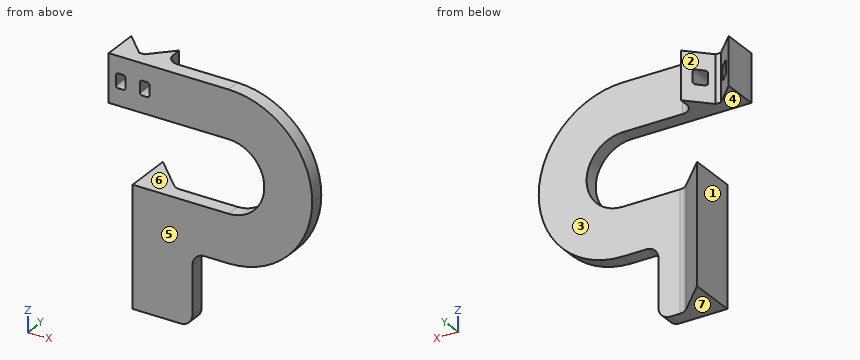
from build123d import *

# Parameters (mm, degrees)
F1_DEPTH = 6
F3_DEPTH = 50
F5_DEPTH = 20
F6_R     = 5
F7_DEPTH = 14.001
F8_R     = 1


with BuildPart() as f1:
    # F0 (on Front) → F1 (new body)
    with BuildSketch(Plane.XZ):
        with BuildLine():
            Line((-10, 15), (8.3772233983, 15))
            ThreePointArc((8.3772233983, 15), (21.2917130661, 29.5803989155), (40, 35))
            Line((40, 35), (-10, 35))
            Line((-10, 35), (-10, 15))
        make_face()
        Polygon((-7, 22), (-7, 25), (-7, 28), (-3, 28), (-3, 25), (-3, 22), align=None, mode=Mode.SUBTRACT)
        Polygon((7, 22), (3, 22), (3, 25), (3, 28), (7, 28), (7, 25), align=None, mode=Mode.SUBTRACT)
        with BuildLine():
            Line((40, -15), (25, -15))
            Line((25, -15), (25, -31.6227766017))
            ThreePointArc((25, -31.6227766017), (32.312255892, -34.1452572187), (40, -35))
            ThreePointArc((40, -35), (64.7487373415, -24.7487373415), (75, 0))
            ThreePointArc((75, 0), (64.7487373415, 24.7487373415), (40, 35))
            ThreePointArc((40, 35), (21.2917130661, 29.5803989155), (8.3772233983, 15))
            Line((8.3772233983, 15), (40, 15))
            ThreePointArc((40, 15), (50.6066017178, 10.6066017178), (55, 0))
            ThreePointArc((55, 0), (50.6066017178, -10.6066017178), (40, -15))
        make_face()
        with BuildLine():
            Line((25, -15), (8.3772233983, -15))
            ThreePointArc((8.3772233983, -15), (15.2512626585, -24.7487373415), (25, -31.6227766017))
            Line((25, -31.6227766017), (25, -15))
        make_face()
        with BuildLine():
            Line((8.3772233983, -15), (0, -15))
            Line((0, -15), (0, -65))
            Line((0, -65), (25, -65))
            Line((25, -65), (25, -35))
            Line((25, -35), (25, -31.6227766017))
            ThreePointArc((25, -31.6227766017), (15.2512626585, -24.7487373415), (8.3772233983, -15))
        make_face()
        with BuildLine():
            ThreePointArc((40, -35), (32.312255892, -34.1452572187), (25, -31.6227766017))
            Line((25, -31.6227766017), (25, -35))
            Line((25, -35), (40, -35))
        make_face()
    extrude(amount=F1_DEPTH)

    # F2 (on face) → F3 (join)
    with BuildSketch(Plane.XY.offset(-15)):
        Polygon((0, 0), (14, 0), (0, 14), align=None)
    extrude(amount=-F3_DEPTH)

    # F4 (on face) → F5 (join, through all)
    with BuildSketch(Plane.XY.offset(35)):
        Polygon((-10, 0), (-1.0710678119, 0), (-10, 8.9289321881), align=None)
        Polygon((1.0710678119, 0), (10, 0), (10, 8.9289321881), align=None)
    extrude(amount=-F5_DEPTH)

    # F6
    f6_edges = [f1.edges().sort_by_distance(p)[0] for p in [
        (25, -3, -35),
        (25, -3, -65),
        (10, 0, 25),
        (14, 0, -40),
    ]]
    fillet(f6_edges, radius=F6_R)

    # F0 (on Front) → F7 (cut, through all)
    with BuildSketch(Plane.XZ):
        Polygon((-7, 28), (-7, 25), (-7, 22), (-3, 22), (-3, 25), (-3, 28), align=None)
        Polygon((3, 25), (3, 22), (7, 22), (7, 25), (7, 28), (3, 28), align=None)
    extrude(amount=-F7_DEPTH, mode=Mode.SUBTRACT)

    # F8
    f8_edges = [f1.edges().sort_by_distance(p)[0] for p in [
        (7, -0.035534, 22),
        (-3, -2.035534, 22),
        (7, -0.035534, 28),
        (-3, -2.035534, 28),
        (-7, -0.035534, 28),
        (3, -2.035534, 28),
        (-7, -0.035534, 22),
        (3, -2.035534, 22),
    ]]
    fillet(f8_edges, radius=F8_R)


solid = f1.part
Input: part model. Units: mm. Frame: model coordinates. Face numbers are marked on the shaded views. A direction names the side the tool comes from. Round coordinates to 2 decimals unless told otherwise and drop trailing zeros. Order: outer loops, then holes, each group sorted by start corner. A loop starts at its lowest first (then second) coordinate and runs counter-clockwise, first axis right, second up. Notation, with made-up numbers: (81, 55.25) - (98, 55.25) arc R15 cw to (98, 74.25) - close; hole circle Ø9 at (-8.5, 83). An arc over 180 degrees is marked (long way). Use a Markdown table: item, result.
1. Access query for the marked faces 1, 2, 3 and 4. Directions: +Z, -Z, +X, -X, +Y, -Y. A direction counts if a zero-diameter tool reaches every point of the face in a straight line with its end or side. Return the directions, or none.
Evaluation:
| item | result |
|---|---|
| face 1 | -Z, -X, +Y, -Y |
| face 2 | +Z, +Y |
| face 3 | +Z, -Z, +X, +Y |
| face 4 | -X, +Y, -Y |
2. Section C-C on z = -57. Return the cut outline in (x, y).
Evaluation:
| item | result |
|---|---|
| outline | (0, -6) - (25, -6) - (25, 0) - (16.07, 0) arc R5 cw to (12.54, 1.46) - (0, 14) - close |
3. Material intervals for probe 1 along Z at (x, y) = (-4, -0.25); probe 2 along Y at (x, z) = (16, 21); probe 3 along Y at (x, z) = (10, -45.5), sorted ascending.
Evaluation:
| item | result |
|---|---|
| probe 1 | 15 to 22, 28 to 35 |
| probe 2 | -6 to 0 |
| probe 3 | -6 to 4 |
4. Section A-A on x = 35.5. Return the cut outline in (y, z), then the cut area to 3 significant figures.
Evaluation:
| item | result |
|---|---|
| outline | (-6, -35) - (0, -35) - (0, -15) - (-6, -15) - close; (-6, 15) - (0, 15) - (0, 35) - (-6, 35) - close |
| area | 240 mm^2 |
5. Section D-D on x = 47.5. Return the cut outline in (y, z).
Evaluation:
| item | result |
|---|---|
| outline | (-6, -34.19) - (0, -34.19) - (0, -12.99) - (-6, -12.99) - close; (-6, 12.99) - (0, 12.99) - (0, 34.19) - (-6, 34.19) - close |
6. First-contact query: pin 1 (2 mm diameter, centred on x = 30.5, z = -36.5, fed in from -Y); pin 2 (4.5 mm diameter, centred on y = -2.5, z = 25.5, fed in from +X); pin 3 (3 mm diameter, centred on y = 6.5, z = 25, fed in from +X); pin 4 (18 mm diameter, centred on x = 39.5, z = -30, fed in from +Y). Flat tips, straight axial feed; report the tip coordinate or a pass-through.
Evaluation:
| item | result |
|---|---|
| pin 1 | through |
| pin 2 | x = 66.16 |
| pin 3 | x = 10 |
| pin 4 | y = 0 |
7. Mould query, pull axis Z, two halves, no side actions, for the marked faces 5, 6 and 7. Classes: +Z half, -Z half, draft (parallel to the pull), parting line (faces both ways), or undercut.
Evaluation:
| item | result |
|---|---|
| face 5 | draft |
| face 6 | undercut |
| face 7 | -Z half |
8. Section B-B on y = -2.5. Return the cut outline in (x, z).
Evaluation:
| item | result |
|---|---|
| outline | (-10, 15) - (40, 15) arc R15 cw to (40, -15) - (0, -15) - (0, -65) - (20, -65) arc R5 ccw to (25, -60) - (25, -40) arc R5 cw to (30, -35) - (40, -35) arc R35 ccw to (40, 35) - (-10, 35) - close; hole (-7, 23) arc R1 ccw to (-6, 22) - (-4, 22) arc R1 ccw to (-3, 23) - (-3, 27) arc R1 ccw to (-4, 28) - (-6, 28) arc R1 ccw to (-7, 27) - close; hole (3, 23) arc R1 ccw to (4, 22) - (6, 22) arc R1 ccw to (7, 23) - (7, 27) arc R1 ccw to (6, 28) - (4, 28) arc R1 ccw to (3, 27) - close |
